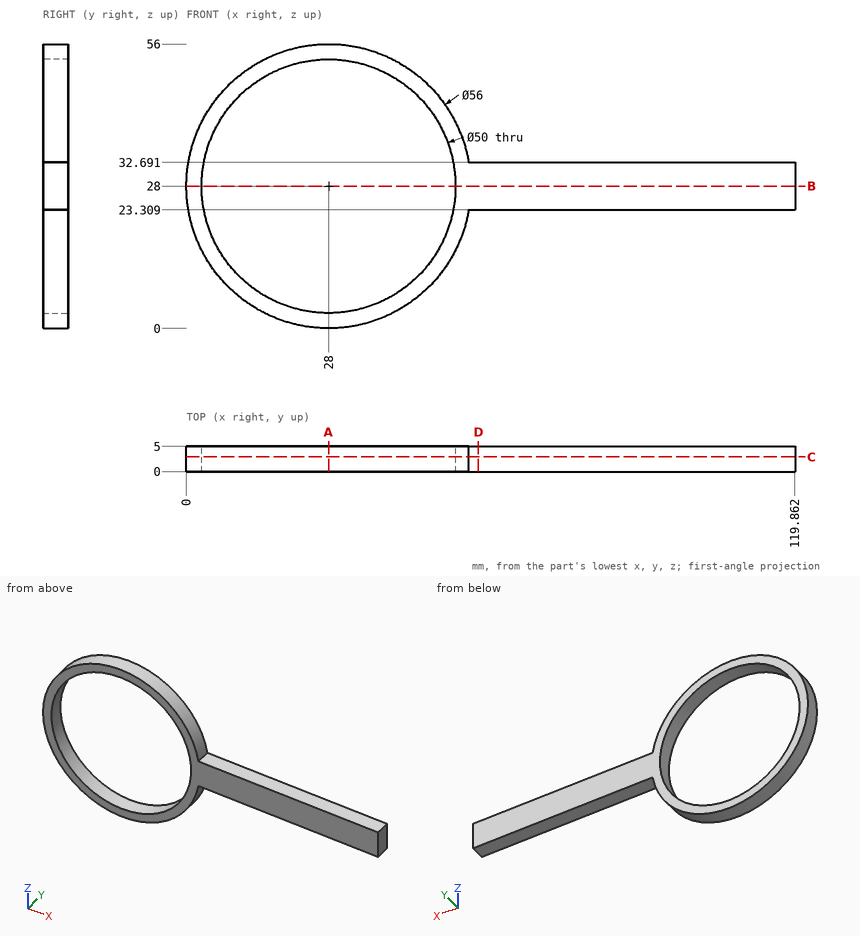
Geometry: see drawing. Coordinates: mm, zero at the bounding-box minimum. Give positions to 0.01 mm unless a question says otherwise; leave off trailing zeros. Write each loop counter-clockwise with the first axis right and the second up, starting at its lowest first coordinate (ties: lowest second). Pieces come first, ordered by that corner, then holes. Notation, with made-up numbers: (19, -22.5) -> (29, -22.5) arc R30 ccw to (29, 11.5) -> close; hole circle Ø5 at (21.5, -12). An arc over 180 degrees is marked (long way). Use one line per item in the form item = value. Start each with the question number.
1) Section query B-B on z = 28. Return the cut outline in (x, y), then the cut area to 3 significant figures.
2) Ray query, probe 1 along X at (y, z) = (3.3, 28); probe 2 along X at (y, z) = (3.5, 11.5); probe 3 along Z at (x, y) = (111, 2.7). Return the intervals inside material, ascending. Write a range as from..to.
3) Pin query (flat end, axial travel): pin 1 (3 mm diameter, centred on x = 64.5, y = 4.5, fed in from +Z); pin 2 (1.5 mm diameter, centred on y = 4, z = 50, fed in from +X). Return the tip coordinate at first contact, or that it passes through.
4) Section query A-A on x = 28. Return the cut outline in (y, z).
5) Section query D-D on x = 57.5. Return the cut outline in (y, z).
6) Section query C-C on y = 2.95. Return the cut outline in (x, z).
Outcome:
q1.outline = (0, 0) -> (3, 0) -> (3, 5) -> (0, 5) -> close; (53, 0) -> (119.86, 0) -> (119.86, 5) -> (53, 5) -> close
q1.area = 349 mm^2
q2.probe_1 = 0..3, 53..119.86
q2.probe_2 = 5.38..9.22, 46.78..50.62
q2.probe_3 = 23.31..32.69
q3.pin_1 = 32.69
q3.pin_2 = 46.23
q4.outline = (0, 0) -> (5, 0) -> (5, 3) -> (0, 3) -> close; (0, 53) -> (5, 53) -> (5, 56) -> (0, 56) -> close
q5.outline = (0, 23.31) -> (5, 23.31) -> (5, 32.69) -> (0, 32.69) -> close
q6.outline = (55.6, 23.31) -> (119.86, 23.31) -> (119.86, 32.69) -> (55.6, 32.69) arc R28 ccw (long way) to start; hole circle Ø50 at (28, 28)
